from build123d import *

# Parameters (mm, degrees)
ESQUISSE12_R        = 1.5
ESQUISSE12_W        = 3
ESQUISSE12_H        = 6
ESQUISSE12_W_2      = 10
ESQUISSE12_H_2      = 3
ESQUISSE12_W_3      = 23
ESQUISSE12_H_3      = 11.8
BOSS_EXTRU_12_DEPTH = 3


with BuildPart() as part:
    # Esquisse12 → Boss.-Extru.12 (new body)
    with BuildSketch(Plane.XY):
        with BuildLine():
            Line((218.080291561, -14.564673514), (164.080291561, -14.564673514))
            ThreePointArc((164.080291561, -14.564673514), (161.958971217, -13.685993857), (161.080291561, -11.564673514))
            Line((161.080291561, -11.564673514), (161.080291561, 27.435326486))
            ThreePointArc((161.080291561, 27.435326486), (161.958971217, 29.55664683), (164.080291561, 30.435326486))
            Line((164.080291561, 30.435326486), (218.080291561, 30.435326486))
            ThreePointArc((218.080291561, 30.435326486), (220.201611904, 29.55664683), (221.080291561, 27.435326486))
            Line((221.080291561, 27.435326486), (221.080291561, -11.564673514))
            ThreePointArc((221.080291561, -11.564673514), (220.201611904, -13.685993857), (218.080291561, -14.564673514))
        make_face()
        with Locations((191.080291561, -10.064673514)):
            Circle(ESQUISSE12_R, mode=Mode.SUBTRACT)
        with Locations((181.580291561, 8.835326486)):
            Circle(ESQUISSE12_R, mode=Mode.SUBTRACT)
        with Locations((181.580291561, 27.835326486)):
            Circle(ESQUISSE12_R, mode=Mode.SUBTRACT)
        with Locations((216.580291561, -2.064673514)):
            Circle(ESQUISSE12_R, mode=Mode.SUBTRACT)
        with Locations((165.580291561, -2.064673514)):
            Circle(ESQUISSE12_R, mode=Mode.SUBTRACT)
        with Locations((165.580291561, -8.564673514)):
            Rectangle(ESQUISSE12_W, ESQUISSE12_H, mode=Mode.SUBTRACT)
        with Locations((173.580291561, -10.064673514)):
            Rectangle(ESQUISSE12_W_2, ESQUISSE12_H_2, mode=Mode.SUBTRACT)
        with Locations((216.580291561, -8.564673514)):
            Rectangle(ESQUISSE12_W, ESQUISSE12_H, mode=Mode.SUBTRACT)
        with Locations((208.580291561, -10.064673514)):
            Rectangle(ESQUISSE12_W_2, ESQUISSE12_H_2, mode=Mode.SUBTRACT)
        with Locations((165.580291561, 4.435326486)):
            Rectangle(ESQUISSE12_W, ESQUISSE12_H, mode=Mode.SUBTRACT)
        with Locations((216.580291561, 4.435326486)):
            Rectangle(ESQUISSE12_W, ESQUISSE12_H, mode=Mode.SUBTRACT)
        with Locations((181.580291561, 18.335326486)):
            Rectangle(ESQUISSE12_W_3, ESQUISSE12_H_3, mode=Mode.SUBTRACT)
    extrude(amount=BOSS_EXTRU_12_DEPTH)


solid = part.part
Here's how the part is built. I have some questions about the finished solid (model axes, mm). Coordinates: 2 decimals unless noted, no trailing zeros. Order: outer loops, then holes, each group sorted by start corner. A loop starts at its lowest first (then second) coordinate and runs counter-clockwise, first axis right, second up. Notation, with made-up numbers: M 5,30 L 60,30 A12 ccw 60,48 Z; hole C 29,56.25 d8. An arc over 180 degrees is marked long. Answer as CSV lines item,"result". Start each with the question number.
1. I want a section at A-A, the plane x = 211.5. Write out the boundary of the cut face in (y, z), and give its area (3 significant figures).
2. I want a section at C-C, the plane x = 177.5. Write out the boundary of the cut face in (y, z), and give its area (3 significant figures).
3. I want a section at B-B, the plane y = 22. Write out the boundary of the cut face in (x, z), and give its area (3 significant figures).
4. We'd pull the mould along X, two halves only. Please class faces 1 (the flat face through (203.58, -10, 1)), 2 (the cylindrical face through (220.225, -13.663, 1.479)), 3 (the flat face through (217, 1.435, 1)): released by +X, released by -X, zero draft, split by the parting line, or undercut.
5. I need wall thicknesses on line 1 (Y direction, x = 174, z = 0.7); line 2 (X direction, y = 2.5, z = 0.9); line 3 (Y direction, x = 208, z = 1.1). Which ranges of each line are inside material? Lowest first, please. Write a range as [from, to].
6. I want a section at D-D, the plane z = 1.1. Count the separate pieces of the cut face and the enclosed holes in it, and give its area (3 significant figures).
7. For pin 1 (4 mm diameter, centred on x = 181.58, y = 8.84, fed in from -Z); pin 2 (2.5 mm diameter, centred on x = 165.58, y = -2.06, fed in from -Z), each with a flat end and sliding along its axis, tell me the tip position at first contact or that it passes through.
Recorded:
1,outline,"M -14.56,0 L -11.56,0 L -11.56,3 L -14.56,3 Z; M -8.56,0 L 30.44,0 L 30.44,3 L -8.56,3 Z"
1,area,"126 mm2"
2,outline,"M -14.56,0 L -11.56,0 L -11.56,3 L -14.56,3 Z; M -8.56,0 L 12.44,0 L 12.44,3 L -8.56,3 Z; M 24.24,0 L 30.44,0 L 30.44,3 L 24.24,3 Z"
2,area,"90.6 mm2"
3,outline,"M 161.08,0 L 170.08,0 L 170.08,3 L 161.08,3 Z; M 193.08,0 L 221.08,0 L 221.08,3 L 193.08,3 Z"
3,area,"111 mm2"
4,face 1,"undercut"
4,face 2,"released by +X"
4,face 3,"undercut"
5,line 1,"y = [-14.56, -11.56], [-8.56, 12.44], [24.24, 30.44]"
5,line 2,"x = [161.08, 164.08], [167.08, 215.08], [218.08, 221.08]"
5,line 3,"y = [-14.56, -11.56], [-8.56, 30.44]"
6,separate pieces,"1"
6,enclosed holes,"12"
6,area,"2,250 mm2"
7,pin 1,"stops at z = 0"
7,pin 2,"passes through"
